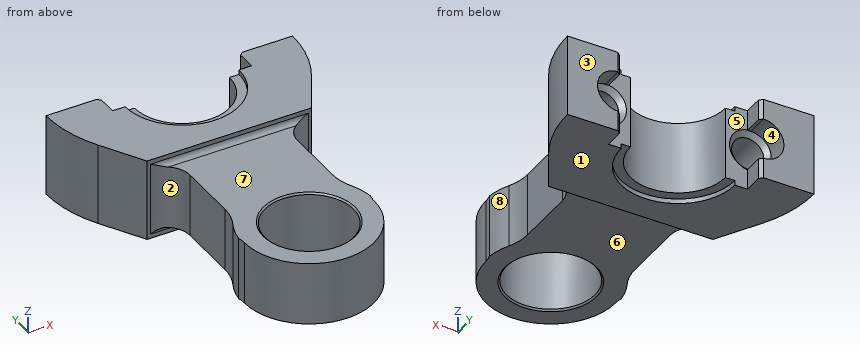
from build123d import *

# Parameters (mm, degrees)
SKETCH_1_R                  = 14
EXTRUDE_1_DEPTH             = 13
CUT_EXTRUDE_1_DEPTH         = 106.812333875
CUT_EXTRUDE_1_DEPTH_BACK    = 106.812333875
SKETCH_2_OUTSIDE_W          = 53.508
SKETCH_2_OUTSIDE_H          = 125.008
CUT_EXTRUDE_2_DEPTH         = 7
CHAMFER_1_SIZE              = 1
CHAMFER_2_SIZE              = 0.5
SKETCH_4_R                  = 18
CUT_EXTRUDE_3_DEPTH         = 1.5
HOLE_WIZARD_M121_AT_2_COUNT = 2
HOLE_WIZARD_M121_AT_2_PITCH = 46


with BuildPart() as part:
    # Эскиз1 → Бобышка-Вытянуть1 (new, symmetric)
    with BuildSketch(Plane.XY):
        with BuildLine():
            Line((33.795797544, -19.463917086), (26, -33))
            Line((26, -33), (25, -33))
            ThreePointArc((25, -33), (19.343145751, -35.343145751), (17, -41))
            Line((17, -41), (17, -60.266799469))
            ThreePointArc((17, -60.266799469), (17.438439597, -63.986723909), (18.72972973, -67.502778077))
            ThreePointArc((18.72972973, -67.502778077), (20.084453039, -70.866913818), (20.840163934, -74.413966902))
            ThreePointArc((20.840163934, -74.413966902), (20.58540569, -75.695845227), (20.5, -77))
            ThreePointArc((20.5, -77), (0, -97.5), (-20.5, -77))
            ThreePointArc((-20.5, -77), (-20.58540569, -75.695845227), (-20.840163934, -74.413966902))
            ThreePointArc((-20.840163934, -74.413966902), (-20.084453039, -70.866913818), (-18.72972973, -67.502778077))
            ThreePointArc((-18.72972973, -67.502778077), (-17.438439597, -63.986723909), (-17, -60.266799469))
            Line((-17, -60.266799469), (-17, -41))
            ThreePointArc((-17, -41), (-19.343145751, -35.343145751), (-25, -33))
            Line((-25, -33), (-26, -33))
            Line((-26, -33), (-33.795797544, -19.463917086))
            ThreePointArc((-33.795797544, -19.463917086), (-37.676492036, -10.073824889), (-39, 0))
            Line((-39, 0), (-22, 0))
            Line((-22, 0), (-22, -7))
            Line((-22, -7), (-15, -7))
            ThreePointArc((-15, -7), (0, -22), (15, -7))
            Line((15, -7), (22, -7))
            Line((22, -7), (22, 0))
            Line((22, 0), (39, 0))
            ThreePointArc((39, 0), (37.676492036, -10.073824889), (33.795797544, -19.463917086))
        make_face()
        with Locations(Location((0, -77, 0), (0, 0, 180))):
            Circle(SKETCH_1_R, mode=Mode.SUBTRACT)
    extrude(amount=EXTRUDE_1_DEPTH, both=True)

    # Эскиз2 outside → Вырез-Вытянуть1 (cut, two sides: drawn at the far end of the back side and taken through both)
    with BuildSketch(Plane(origin=(0, 0, 0), x_dir=(0, 0, -1), z_dir=(1, 0, 0)).offset(-CUT_EXTRUDE_1_DEPTH_BACK)):
        with Locations((0, -48.75)):
            Rectangle(SKETCH_2_OUTSIDE_W, SKETCH_2_OUTSIDE_H)
        with BuildLine():
            Line((13, 0), (-13, 0))
            Line((-13, 0), (-13, -33))
            Line((-13, -33), (-11.6, -33))
            ThreePointArc((-11.6, -33), (-10.46862915, -33.46862915), (-10, -34.6))
            Line((-10, -34.6), (-10, -97.5))
            Line((-10, -97.5), (10, -97.5))
            Line((10, -97.5), (10, -34.6))
            ThreePointArc((10, -34.6), (10.46862915, -33.46862915), (11.6, -33))
            Line((11.6, -33), (13, -33))
            Line((13, -33), (13, 0))
        make_face(mode=Mode.SUBTRACT)
    extrude(amount=CUT_EXTRUDE_1_DEPTH + CUT_EXTRUDE_1_DEPTH_BACK, mode=Mode.SUBTRACT)

    # Эскиз3 → Вырез-Вытянуть2 (cut)
    with BuildSketch(Plane(origin=(0, 0, 0), x_dir=(1, 0, 0), z_dir=(0, 1, 0))):
        with BuildLine():
            Line((23, 6.5), (22, 6.5))
            Line((22, 6.5), (22, -6.5))
            Line((22, -6.5), (23, -6.5))
            ThreePointArc((23, -6.5), (29.5, 0), (23, 6.5))
        make_face()
        with BuildLine():
            Line((-22, 6.5), (-22, -6.5))
            Line((-22, -6.5), (-23, -6.5))
            ThreePointArc((-23, -6.5), (-29.5, 0), (-23, 6.5))
            Line((-23, 6.5), (-22, 6.5))
        make_face()
    extrude(amount=-CUT_EXTRUDE_2_DEPTH, mode=Mode.SUBTRACT)

    # Фаска1
    chamfer_1_edges = [part.edges().sort_by_distance(p)[0] for p in [
        (22, 0, -9.75),
        (22, 0, 9.75),
        (-22, 0, 9.75),
        (-22, 0, -9.75),
    ]]
    chamfer(chamfer_1_edges, length=CHAMFER_1_SIZE)

    # Фаска2
    chamfer_2_edges = [part.edges().sort_by_distance(p)[0] for p in [
        (14, -77, -10),
        (14, -77, 10),
    ]]
    chamfer(chamfer_2_edges, length=CHAMFER_2_SIZE)

    # Эскиз4 → Вырез-Вытянуть3 (cut)
    with BuildSketch(Plane.XY.offset(13)):
        with Locations((0, -7)):
            Circle(SKETCH_4_R)
    cut_extrude_3 = extrude(amount=-CUT_EXTRUDE_3_DEPTH, mode=Mode.SUBTRACT)

    # Зеркальное отражение1: Вырез-Вытянуть3 across plane
    add(cut_extrude_3.mirror(Plane.XY), mode=Mode.SUBTRACT)

    # Эскиз6 → Отверстие обработанное метчиком M121 (revolve, cut)
    with BuildSketch(Plane(origin=(-23, -7, 0), x_dir=(0, 0, 1), z_dir=(1, 0, 0))):
        Polygon((0, 0), (0, 19.944486373), (5.1, 17), (5.1, 1.6), (6.7, 0), align=None)
    hole_wizard_m121 = revolve(axis=Axis((-23, -0.65, 0), (0, -1, 0)), mode=Mode.SUBTRACT)

    # Отверстие обработанное метчиком M121 at 2: Отверстие обработанное метчиком M121 ×2
    with Locations(*[(i * HOLE_WIZARD_M121_AT_2_PITCH, 0, 0) for i in range(1, HOLE_WIZARD_M121_AT_2_COUNT)]):
        add(hole_wizard_m121, mode=Mode.SUBTRACT)


solid = part.part
Geometry: final body of the model. Coordinates: model frame, mm. Face numbers are marked on the shaded views. A direction names the side the tool comes from. Give positions to 0.01 mm unless a question says otherwise; leave off trailing zeros. Loops run counter-clockwise (first coordinate to the right, second up) from the corner with the lowest first, then second, coordinate; pieces in that order, holes last. Notation, with made-up numbers: (0.5, 20) -> (31.5, 20) arc R9 cw to (31.5, 33) -> close; hole circle Ø11 at (29, 2.25). An arc over 180 degrees is marked (long way). Put each result on its own line as item: value.
1. Pin query (flat end, axial travel): P1, Ø12, axis at x = -21.5, z = 3.5, coming from the +Y side; P2, Ø9, axis at x = -23, z = 0, coming from the -Y side; P3, Ø1.8, axis at y = -5.5, z = -9.5, coming from the -X side; P4, Ø3, axis at x = -10.5, z = -1.5, coming from the -Y side. Return the tip coordinate at first contact, or that it passes through.
Taken from the geometry:
P1: stops at y = 0
P2: stops at y = -85.83
P3: stops at x = -38.73
P4: stops at y = -95.42
2. Cut plane A-A (x = 0). Return the cut outline in (y, z).
Taken from the geometry:
outline: (-97.5, -10) -> (-91.5, -10) -> (-91, -9.5) -> (-91, 9.5) -> (-91.5, 10) -> (-97.5, 10) -> close; (-63, -9.5) -> (-62.5, -10) -> (-34.6, -10) arc R1.6 cw to (-33, -11.6) -> (-33, -13) -> (-25, -13) -> (-25, -11.5) -> (-22, -11.5) -> (-22, 11.5) -> (-25, 11.5) -> (-25, 13) -> (-33, 13) -> (-33, 11.6) arc R1.6 cw to (-34.6, 10) -> (-62.5, 10) -> (-63, 9.5) -> close
3. Set-up query: the marked faces 4, 5, 6, 7 and 8. Return all of +Z, -Z, +X, -X, +Y, -Y with unobstructed straight access to the full face (end or side cutting, diameter ignored); none if empty.
Taken from the geometry:
face 4: +Y
face 5: +Z, -Z, +Y
face 6: -Z, +X, -X, -Y
face 7: +Z, +X, -X, -Y
face 8: +Z, -Z, +X
4. Cut plane B-B (y = -46). Return the cut outline in (x, z).
Taken from the geometry:
outline: (-17, -10) -> (17, -10) -> (17, 10) -> (-17, 10) -> close
5. Pull-direction query (Y, two-part tool) for the marked faces 1, 2 and 3; classes: released by +Y, released by -Y, zero draft, split by the parting line, or undercut.
Taken from the geometry:
face 1: zero draft
face 2: undercut
face 3: released by +Y
6. Ray query, line 1 along Z through (x, y) = (23, -15.5); line 2 along X through (y, z) = (-76.5, -7.25); line 3 along X through (y, z) = (-14.5, 0). Return the intervals inside material, ascending. Write a range as [from, to].
Taken from the geometry:
line 1: z = [-13, -5.1], [5.1, 13]
line 2: x = [-20.51, -13.99], [13.99, 20.51]
line 3: x = [-36.2, -28.1], [-17.9, -12.99], [12.99, 17.9], [28.1, 36.2]
